The model under review builds one solid part; all positions refer to its coordinate system, in mm. Round coordinates to 2 decimals unless told otherwise and drop trailing zeros. Write each loop counter-clockwise with the first axis right and the second up, starting at its lowest first coordinate (ties: lowest second). Pieces come first, ordered by that corner, then holes.
Item 1: Clearance check with flat-ended pins moving along their axes: pin 1 Ø3.5 at (x, z) = (19.45, -19.45) entering from +Y; pin 2 Ø5.5 at (x, z) = (12.37, 12.37) entering from -Y; pin 3 Ø1 at (y, z) = (3.5, -17) entering from -X; pin 4 Ø1.5 at (x, y) = (-10.5, 4) entering from -Z. State where each tip first meets the part, or that it passes through.
Item 2: Add section A-A (x = 0). Give the boundary of the cut face in (y, z), plus the area to 3 significant figures.
Item 3: Draft analysis for pull direction X (two halves, no side actions). For faces 1 (the face through (21, 2, 0)), 2 (the face through (23.07, 2.46, -22.89)), 3 (the face through (-19.38, 2.46, 11.87)), 4 (the face through (11.87, 2.46, 19.38)), state which applies: +X half, -X half, draft (parallel to the pull), parting line (faces both ways), or undercut.
Item 4: Add section B-B (z = -0.5). Give the boundary of the cut face in (x, y).
Item 5: To check wall thickness, follow L1, parallel to X at y = 3.35, z = 18.5; L2, parallel to Z at x = -3.5, y = 3.6. State the ranges of each line that lie inside material, in increasing order.
Item 6: Add section C-C (y = 0.65). State how many separate pieces and enclosed holes the cut face has, plus the area to 3 significant figures.
```python
from build123d import *

# Parameters (mm, degrees)
SKETCH_1_R      = 13.5
SKETCH_1_R_2    = 2.15
EXTRUDE_1_DEPTH = 5


with BuildPart() as part:
    # ｽｹｯﾁ1 → ﾎﾞｽ - 押し出し1 (new body)
    with BuildSketch(Plane(origin=(0, 0, 0), x_dir=(1, 0, 0), z_dir=(0, 1, 0))):
        with BuildLine():
            ThreePointArc((19.507056212, -7.776551803), (21, 0), (19.507056212, 7.776551803))
            ThreePointArc((19.507056212, 7.776551803), (19.398069264, 11.924552334), (22.006829374, 15.151339784))
            ThreePointArc((22.006829374, 15.151339784), (22.980970389, 22.980970389), (15.151339784, 22.006829374))
            ThreePointArc((15.151339784, 22.006829374), (11.924552334, 19.398069264), (7.776551803, 19.507056212))
            ThreePointArc((7.776551803, 19.507056212), (0, 21), (-7.776551803, 19.507056212))
            ThreePointArc((-7.776551803, 19.507056212), (-11.924552334, 19.398069264), (-15.151339784, 22.006829374))
            ThreePointArc((-15.151339784, 22.006829374), (-22.980970389, 22.980970389), (-22.006829374, 15.151339784))
            ThreePointArc((-22.006829374, 15.151339784), (-19.398069264, 11.924552334), (-19.507056212, 7.776551803))
            ThreePointArc((-19.507056212, 7.776551803), (-21, 0), (-19.507056212, -7.776551803))
            ThreePointArc((-19.507056212, -7.776551803), (-19.398069264, -11.924552334), (-22.006829374, -15.151339784))
            ThreePointArc((-22.006829374, -15.151339784), (-22.980970389, -22.980970389), (-15.151339784, -22.006829374))
            ThreePointArc((-15.151339784, -22.006829374), (-11.924552334, -19.398069264), (-7.776551803, -19.507056212))
            ThreePointArc((-7.776551803, -19.507056212), (0, -21), (7.776551803, -19.507056212))
            ThreePointArc((7.776551803, -19.507056212), (11.924552334, -19.398069264), (15.151339784, -22.006829374))
            ThreePointArc((15.151339784, -22.006829374), (22.980970389, -22.980970389), (22.006829374, -15.151339784))
            ThreePointArc((22.006829374, -15.151339784), (19.398069264, -11.924552334), (19.507056212, -7.776551803))
        make_face()
        with Locations(Location((0, 0, 0), (0, 0, 270))):
            Circle(SKETCH_1_R, mode=Mode.SUBTRACT)
        with Locations(Location((12.374368671, 12.374368671, 0), (0, 0, 270))):
            Circle(SKETCH_1_R_2, mode=Mode.SUBTRACT)
        with Locations(Location((12.374368671, -12.374368671, 0), (0, 0, 270))):
            Circle(SKETCH_1_R_2, mode=Mode.SUBTRACT)
        with Locations(Location((-12.374368671, -12.374368671, 0), (0, 0, 270))):
            Circle(SKETCH_1_R_2, mode=Mode.SUBTRACT)
        with Locations(Location((-12.374368671, 12.374368671, 0), (0, 0, 270))):
            Circle(SKETCH_1_R_2, mode=Mode.SUBTRACT)
        with Locations(Location((19.445436483, 19.445436483, 0), (0, 0, 270))):
            Circle(SKETCH_1_R_2, mode=Mode.SUBTRACT)
        with Locations(Location((19.445436483, -19.445436483, 0), (0, 0, 270))):
            Circle(SKETCH_1_R_2, mode=Mode.SUBTRACT)
        with Locations(Location((-19.445436483, -19.445436483, 0), (0, 0, 270))):
            Circle(SKETCH_1_R_2, mode=Mode.SUBTRACT)
        with Locations(Location((-19.445436483, 19.445436483, 0), (0, 0, 270))):
            Circle(SKETCH_1_R_2, mode=Mode.SUBTRACT)
    extrude(amount=EXTRUDE_1_DEPTH)


solid = part.part
```
Numbers:
1. pin 1: passes through
1. pin 2: stops at y = 0
1. pin 3: stops at x = -24.05
1. pin 4: stops at z = -19.21
2. outline: (0, -21) - (5, -21) - (5, -13.5) - (0, -13.5) - close; (0, 13.5) - (5, 13.5) - (5, 21) - (0, 21) - close
2. area: 75.0 mm2
3. face 1: +X half
3. face 2: undercut
3. face 3: -X half
3. face 4: undercut
4. outline: (-20.99, 0) - (-13.49, 0) - (-13.49, 5) - (-20.99, 5) - close; (13.49, 0) - (20.99, 0) - (20.99, 5) - (13.49, 5) - close
5. L1: x = -24.36 to -21.38, -17.51 to 17.51, 21.38 to 24.36
5. L2: z = -20.71 to -13.04, 13.04 to 20.71
6. separate pieces: 1
6. enclosed holes: 9
6. area: 1,130 mm2
